Autodesk Inventor part; units mm, degrees
ref_plane "YZ Plane" through (0, 0, 0) normal (1, 0, 0) x (0, 1, 0)
ref_plane "XZ Plane" through (0, 0, 0) normal (0, 1, 0) x (-1, 0, 0)
ref_plane "XY Plane" through (0, 0, 0) normal (0, 0, 1) x (1, 0, 0)
sketch "Sketch1" plane through (0, 0, 0) normal (0, 0, 1) x (1, 0, 0)
  line L0 (-15, 57.0488) -> (55, 57.0488)
  line L1 (-15, 12.0488) -> (-15, 57.0488)
  line L2 (55, 12.0488) -> (-15, 12.0488)
  line L3 (55, 57.0488) -> (55, 12.0488)
  line L4 (-17, 59.0488) -> (57, 59.0488)
  line L5 (57, 59.0488) -> (57, 10.0488)
  line L6 (57, 10.0488) -> (-17, 10.0488)
  line L7 (-17, 10.0488) -> (-17, 59.0488)
  point P0 (0, 0)
  dimension "d0" = 74
  dimension "d1" = 49
  dimension "d2" = 2
  dimension "d3" = 2
extrude "Extrusion1" add sketch "Sketch1" along normal blind 27
sketch "Sketch2" plane through (0, 0, 27) normal (0, 0, 1) x (1, 0, 0)
  line L0 (57, 59.0488) -> (-17, 59.0488)
  line L1 (-17, 59.0488) -> (57, 59.0488)
  line L2 (57, 59.0488) -> (57, 10.0488)
  line L3 (57, 10.0488) -> (-17, 10.0488)
  line L4 (-17, 10.0488) -> (-17, 59.0488)
  point P0 (0, 0)
extrude "Extrusion2" add sketch "Sketch2" along normal blind 3
sketch "Sketch3" plane through (0, 0, 30) normal (0, 0, 1) x (1, 0, 0)
  circle A0 centre (-11, 20.0488) radius 3
  line L0 (-17, 10.0488) -> (57, 10.0488)
  line L1 (-17, 59.0488) -> (-17, 10.0488)
  point P0 (0, 0)
  dimension "d8" = 6
  dimension "d9" = 10
  dimension "d10" = 6
extrude "Extrusion3" cut sketch "Sketch3" against normal up to next
fillet "Fillet1" radius 2 8 edges at (57, 34.5488, 30) (20, 59.0488, 30) (57, 59.0488, 15) (57, 10.0488, 15) (-17, 59.0488, 15) (-17, 34.5488, 30) (-17, 10.0488, 15) (20, 10.0488, 30)
properties part number "Extrusion"
Input: part model. Units: mm. Frame: model coordinates. A direction names the side the tool comes from. Give positions to 0.01 mm unless a question says otherwise; leave off trailing zeros. Write each loop counter-clockwise with the first axis right and the second up, starting at its lowest first coordinate (ties: lowest second). Pieces come first, ordered by that corner, then holes. Notation, with made-up numbers: M 19.25,-4 L 45.25,-4 A19 cw 45.25,25 Z; hole C -11,-22.75 d6. An arc over 180 degrees is marked long. Write item = value, one per line. Start each with the question number.
1) First-contact query: pin 1 Ø12 at (x, y) = (-8.5, 50.5) entering from -Z. Flat tip, straight axial feed; report the tip coordinate or a pass-through.
2) Cut plane D-D on y = 50. Return the cut outline in (x, z).
3) Cut plane B-B on y = 19. Return the cut outline in (x, z), then the cut area to 3 significant figures.
4) Material intervals for line 1 along Y through (x, z) = (-11, 27.85); line 2 along X through (y, z) = (55, 14.75); line 3 along Y through (x, z) = (8.5, 15), sorted ascending. Write a range as [from, to].
5) Cut plane C-C on z = 12.25. Return the cut outline in (x, y), then the cut area to 3 significant figures.
6) Draft query along Y for faces 3 (the flat face through (20, 35, 27)), 4 (the cylindrical face through (19.51, 58.447, 29.43)), 5 (the cylindrical face through (56.43, 34.23, 29.4)). Return one class per face: +Y half, -Y half, draft (parallel to the pull), parting line (faces both ways), or undercut.
7) Reachability of faces 1 (the flat face through (55, 35, 13)), 2 (the cylindrical face through (-16.43, 10.65, 14.2)) from +Z, -Z, +X, -X, +Y, -Y: full face, straight path, thin tool, end or side. Return the list, or none.
8) Cut plane A-A on x = -11. Return the cut outline in (y, z), then the cut area to 3 significant figures.
Solved:
q1.pin_1 = 27
q2.outline = M -17,0 L -15,0 L -15,27 L 55,27 L 55,0 L 57,0 L 57,28 A2 ccw 55,30 L -15,30 A2 ccw -17,28 Z
q3.outline = M -17,0 L -15,0 L -15,27 L -13.81,27 L -13.81,30 L -15,30 A2 ccw -17,28 Z; M -8.19,27 L 55,27 L 55,0 L 57,0 L 57,28 A2 ccw 55,30 L -8.19,30 Z
q3.area = 311 mm2
q4.line_1 = [10.05, 17.05], [23.05, 59.05]
q4.line_2 = [-17, -15], [55, 57]
q4.line_3 = [10.05, 12.05], [57.05, 59.05]
q5.outline = M -17,12.05 A2 ccw -15,10.05 L 55,10.05 A2 ccw 57,12.05 L 57,57.05 A2 ccw 55,59.05 L -15,59.05 A2 ccw -17,57.05 Z; hole M -15,12.05 L 55,12.05 L 55,57.05 L -15,57.05 Z
q5.area = 473 mm2
q6.face_3 = undercut
q6.face_4 = +Y half
q6.face_5 = draft
q7.face_1 = -Z
q7.face_2 = +Z, -Z, -X, -Y
q8.outline = M 10.05,0 L 12.05,0 L 12.05,27 L 17.05,27 L 17.05,30 L 12.05,30 A2 ccw 10.05,28 Z; M 23.05,27 L 57.05,27 L 57.05,0 L 59.05,0 L 59.05,28 A2 ccw 57.05,30 L 23.05,30 Z
q8.area = 235 mm2
